from build123d import *

# Parameters (mm, degrees)
F1_DEPTH = 7.112
F2_R     = 3.0734


with BuildPart() as f1:
    # F0 (on Front) → F1 (new body)
    with BuildSketch(Plane.XZ):
        with BuildLine():
            ThreePointArc((-5.258809, -5.404494), (0.123873, -0.021812), (5.506555, -5.404494))
            Line((5.506555, -5.404494), (5.506555, 1.758267))
            Line((5.506555, 1.758267), (5.506555, 5.966515))
            Line((5.506555, 5.966515), (5.506555, 8.921028))
            ThreePointArc((5.506555, 8.921028), (0.123873, 14.30371), (-5.258809, 8.921028))
            Line((-5.258809, 8.921028), (-5.258809, 2.41463))
            Line((-5.258809, 2.41463), (-5.258809, -5.404494))
        make_face()
        with BuildLine():
            Line((-5.258809, -5.404494), (5.506555, -5.404494))
            ThreePointArc((5.506555, -5.404494), (0.123873, -0.021812), (-5.258809, -5.404494))
        make_face()
        with BuildLine():
            ThreePointArc((-5.258809, -5.404494), (0.123873, -10.787176), (5.506555, -5.404494))
            Line((5.506555, -5.404494), (-5.258809, -5.404494))
        make_face()
        with BuildLine():
            ThreePointArc((-5.258809, -31.284998), (0.123873, -36.66768), (5.506555, -31.284998))
            Line((5.506555, -31.284998), (5.506555, -5.404494))
            ThreePointArc((5.506555, -5.404494), (0.123873, -10.787176), (-5.258809, -5.404494))
            Line((-5.258809, -5.404494), (-5.258809, -12.387301))
            Line((-5.258809, -12.387301), (-5.258809, -31.284998))
        make_face()
    extrude(amount=F1_DEPTH)

    # F2
    f2_edges = [f1.edges().sort_by_distance(p)[0] for p in [
        (5.506555, -7.112, -11.181985),
        (5.506555, 0, -11.181985),
        (-5.258809, 0, -11.181985),
        (-5.258809, -7.112, -11.181985),
        (0.123873, 0, 14.30371),
        (0.123873, -7.112, 14.30371),
        (0.123873, 0, -36.66768),
        (0.123873, -7.112, -36.66768),
    ]]
    fillet(f2_edges, radius=F2_R)


solid = f1.part
Verification items for the finished model (mm, model axes). Give positions to 0.01 mm unless a question says otherwise; leave off trailing zeros. Write each loop counter-clockwise with the first axis right and the second up, starting at its lowest first coordinate (ties: lowest second). Pieces come first, ordered by that corner, then holes.
(1) Gauge pin test, flat ends, axial feed: pin 1 (3 mm diameter, centred on x = -3.5, y = -3, fed in from -Z); pin 2 (1.5 mm diameter, centred on x = 2.5, y = -4, fed in from -Z); pin 3 (1 mm diameter, centred on x = 1, y = -2, fed in from -Z). Record the tip position at first contact, or that the pin passes through.
(2) Material ranges on line 1 (X direction, y = -3, z = -28); line 2 (X direction, y = -1, z = -22); line 3 (Z direction, x = -0.5, y = -6.25), recorded low to high.
(3) Cross-section at A-A (z = -28). Enter the section's corners in (x, y), plus the area to 3 significant figures.
(4) Mould release check, pull along Y, two halves, no side actions. Record for faces 1 (the face through (0.006, -3.549, -36.666)), 2 (the face through (4.63, -0.924, -10.901)), 3 (the face through (4.63, -6.19, -10.9)): +Y half, -Y half, draft (parallel to the pull), parting line (faces both ways), or undercut.
Worked out:
1. pin 1: stops at z = -36.23
1. pin 2: stops at z = -36.42
1. pin 3: stops at z = -36.56
2. line 1: x = -5.26 to 5.51
2. line 2: x = -4.45 to 4.7
2. line 3: z = -35.68 to 13.32
3. outline: (-5.26, -4.04) arc R3.07 ccw to (-2.19, -7.11) - (2.43, -7.11) arc R3.07 ccw to (5.51, -4.04) - (5.51, -3.07) arc R3.07 ccw to (2.43, 0) - (-2.19, 0) arc R3.07 ccw to (-5.26, -3.07) - close
3. area: 68.5 mm2
4. face 1: draft
4. face 2: +Y half
4. face 3: -Y half
